Here's how the part is built. I have some questions about the finished solid (model axes, mm). Face numbers are marked on the shaded views. A direction names the side the tool comes from. Give positions to 0.01 mm unless a question says otherwise; leave off trailing zeros. Loops run counter-clockwise (first coordinate to the right, second up) from the corner with the lowest first, then second, coordinate; pieces in that order, holes last. Notation, with made-up numbers: (-37, -11) - (-27, -11) arc R16 cw to (-27, 20) - close; hole circle Ø5 at (68, 80.25). An arc over 180 degrees is marked (long way). One line per item, written item: value. Start each with the question number.
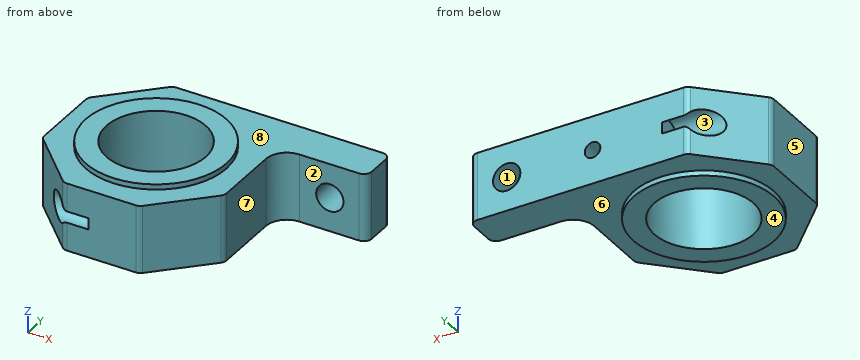
```python
from build123d import *

# Parameters (mm, degrees)
SKETCH1_R           = 19.05
BOSS_EXTRUDE1_DEPTH = 13
FILLET1_R           = 8
FILLET2_R           = 3
SKETCH2_R           = 27
SKETCH2_R_2         = 19.05
BOSS_EXTRUDE2_DEPTH = 15
SKETCH3_R           = 5
CUT_EXTRUDE1_DEPTH  = 30
SKETCH4_R           = 5.25
SKETCH4_R_2         = 3
CUT_EXTRUDE2_DEPTH  = 15


with BuildPart() as part:
    # Sketch1 → Boss-Extrude1 (new body, symmetric)
    with BuildSketch(Plane.XY):
        Polygon((14.497474683, 35), (0, 35), (-14.497474683, 35), (-35, 14.497474683), (-35, -14.497474683), (-14.497474683, -35), (14.497474683, -35), (35, -14.497474683), (35, 20), (69, 20), (69, 35), align=None)
        Circle(SKETCH1_R, mode=Mode.SUBTRACT)
    extrude(amount=BOSS_EXTRUDE1_DEPTH, both=True)

    # Fillet1
    fillet1_edges = [part.edges().sort_by_distance(p)[0] for p in [
        (35, 20, 0),
    ]]
    fillet(fillet1_edges, radius=FILLET1_R)

    # Fillet2
    fillet2_edges = [part.edges().sort_by_distance(p)[0] for p in [
        (69, 35, 0),
        (69, 20, 0),
        (35, -14.497474683, 0),
        (14.497474683, -35, 0),
        (-14.497474683, -35, 0),
        (-35, -14.497474683, 0),
        (-35, 14.497474683, 0),
        (-14.497474683, 35, 0),
    ]]
    fillet(fillet2_edges, radius=FILLET2_R)

    # Sketch2 → Boss-Extrude2 (add, symmetric)
    with BuildSketch(Plane.XY):
        Circle(SKETCH2_R)
        Circle(SKETCH2_R_2, mode=Mode.SUBTRACT)
    extrude(amount=BOSS_EXTRUDE2_DEPTH, both=True)

    # Sketch3 → Cut-Extrude1 (cut)
    with BuildSketch(Plane.ZY.offset(35)):
        with Locations((0, -30.5)):
            Circle(SKETCH3_R)
        with Locations((0, 30.5)):
            Circle(SKETCH3_R)
    extrude(amount=-CUT_EXTRUDE1_DEPTH, mode=Mode.SUBTRACT)

    # Sketch4 → Cut-Extrude2 (cut)
    with BuildSketch(Plane(origin=(0, 35, 0), x_dir=(1, 0, 0), z_dir=(0, 1, 0))):
        with Locations((54.75, 0)):
            Circle(SKETCH4_R)
        with Locations((21.75, 0)):
            Circle(SKETCH4_R_2)
    extrude(amount=-CUT_EXTRUDE2_DEPTH, mode=Mode.SUBTRACT)


solid = part.part
```
(1) If we mould it in two halves opening along Z, with no side actions, what happens to the marked faces 1, 2, 3 and 4? For each: pulls with the +Z half, pulls with the -Z half, needs draft (parallel to the pull), parting line crosses it, or undercut.
(2) If we section it at D-D on x = 54.75: List the corners of the cut face in (y, z) for me, plus the area to 4 significant figures.
(3) If we section it at A-A on y = 0: List the corners of the cut face in (x, z) for me, plus the area to 3 significant figures.
(4) Please list where these lines run through material, in increasing order: probe 1 along X at (y, z) = (30, 0); probe 2 along Z at (x, y) = (-17, -30.5); probe 3 along X at (y, z) = (28.5, 2.5). Write a range as from..to.
(5) If we section it at C-C on y = 30.5: List the corners of the cut face in (x, z) for me.
(6) For the marked faces 5, 6, 7 and 8, which set-ups out of +Z, -Z, +X, -X, +Y, -Y let a thin tool reach every point of the face, with its end or its side?
(7) Will these pins go through, and if not, where does the flat tip stop? pin 1 (10 mm diameter, centred on y = -10.5, z = -12, fed in from +X); pin 2 (10 mm diameter, centred on y = 20.5, z = 3, fed in from -X); pin 3 (9.5 mm diameter, centred on x = 21.75, z = 0, fed in from -Y); pin 4 (12 mm diameter, centred on x = 12.5, y = 12, fed in from +Z).
Found:
1. face 1: undercut
1. face 2: needs draft
1. face 3: undercut
1. face 4: pulls with the -Z half
2. outline: (20, -13) - (35, -13) - (35, -5.25) - (20, -5.25) - close; (20, 5.25) - (35, 5.25) - (35, 13) - (20, 13) - close
2. area: 232.5 mm^2
3. outline: (-35, -13) - (-27, -13) - (-27, -15) - (-19.05, -15) - (-19.05, 15) - (-27, 15) - (-27, 13) - (-35, 13) - close; (19.05, -15) - (27, -15) - (27, -13) - (35, -13) - (35, 13) - (27, 13) - (27, 15) - (19.05, 15) - close
3. area: 893 mm^2
4. probe 1: -5..18.75, 24.75..49.5, 60..69
4. probe 2: -13..-5, 5..13
4. probe 3: -5..20.09, 23.41..50.13, 59.37..69
5. outline: (-19, -13) - (69, -13) - (69, 13) - (-19, 13) - (-19, 5) - (-5, 5) - (-5, -5) - (-19, -5) - close; hole circle Ø6 at (21.75, 0); hole circle Ø10.5 at (54.75, 0)
6. face 5: +Z, -Z, -X, +Y, -Y
6. face 6: -Z
6. face 7: +Z, -Z, +X, -Y
6. face 8: +Z
7. pin 1: x = 35
7. pin 2: x = -34
7. pin 3: y = -32.5
7. pin 4: z = 15
